Geometry check sheet. Reference: the model listing, model coordinates, mm. A direction names the side the tool comes from. Coordinates: 2 decimals unless noted, no trailing zeros. Loops run counter-clockwise (first coordinate to the right, second up) from the corner with the lowest first, then second, coordinate; pieces in that order, holes last.
from build123d import *

# Parameters (mm, degrees)
EXTRUDE_1_DEPTH     = 2
CUT_EXTRUDE_1_REACH = 72.175
SKETCH_2_R          = 1.3
CUT_EXTRUDE_2_REACH = 72.175
SKETCH_3_R          = 1.3
CUT_EXTRUDE_3_REACH = 72.175


with BuildPart() as part:
    # 草图1 → 凸台-拉伸1 (new body)
    with BuildSketch(Plane.XZ.offset(19.39)):
        Polygon((-51.8, -40.295836944), (-44.795836944, -47.3), (37.795836944, -47.3), (44.8, -40.295836944), (44.8, 27.295836944), (37.795836944, 34.3), (-44.795836944, 34.3), (-51.8, 27.295836944), align=None)
    extrude(amount=EXTRUDE_1_DEPTH)

    # 草图2 → 切除-拉伸1 (cut, up to next)
    with BuildSketch(Plane.XZ.offset(21.39), mode=Mode.PRIVATE) as cut_extrude_1_sk1:
        with Locations(Location((-39.011567772, -24.5, 0), (0, 0, 270))):
            Circle(SKETCH_2_R)
    cut_extrude_1_tool1 = extrude(cut_extrude_1_sk1.sketch, amount=-CUT_EXTRUDE_1_REACH, mode=Mode.PRIVATE) & part.part
    # 草图2 → 切除-拉伸1 (cut, up to next)
    with BuildSketch(Plane.XZ.offset(21.39), mode=Mode.PRIVATE) as cut_extrude_1_sk2:
        with Locations(Location((19, -24.5, 0), (0, 0, 270))):
            Circle(SKETCH_2_R)
    cut_extrude_1_tool2 = extrude(cut_extrude_1_sk2.sketch, amount=-CUT_EXTRUDE_1_REACH, mode=Mode.PRIVATE) & part.part
    # 草图2 → 切除-拉伸1 (cut, up to next)
    with BuildSketch(Plane.XZ.offset(21.39), mode=Mode.PRIVATE) as cut_extrude_1_sk3:
        with Locations(Location((-39.011567772, 24.535212594, 0), (0, 0, 270))):
            Circle(SKETCH_2_R)
    cut_extrude_1_tool3 = extrude(cut_extrude_1_sk3.sketch, amount=-CUT_EXTRUDE_1_REACH, mode=Mode.PRIVATE) & part.part
    # 草图2 → 切除-拉伸1 (cut, up to next)
    with BuildSketch(Plane.XZ.offset(21.39), mode=Mode.PRIVATE) as cut_extrude_1_sk4:
        with Locations(Location((19, 24.535212594, 0), (0, 0, 270))):
            Circle(SKETCH_2_R)
    cut_extrude_1_tool4 = extrude(cut_extrude_1_sk4.sketch, amount=-CUT_EXTRUDE_1_REACH, mode=Mode.PRIVATE) & part.part
    add(cut_extrude_1_tool1.solids().sort_by_distance((-39.011568, -21.39, -24.5))[0], mode=Mode.SUBTRACT)
    add(cut_extrude_1_tool2.solids().sort_by_distance((19, -21.39, -24.5))[0], mode=Mode.SUBTRACT)
    add(cut_extrude_1_tool3.solids().sort_by_distance((-39.011568, -21.39, 24.535213))[0], mode=Mode.SUBTRACT)
    add(cut_extrude_1_tool4.solids().sort_by_distance((19, -21.39, 24.535213))[0], mode=Mode.SUBTRACT)

    # 草图3 → 切除-拉伸2 (cut, up to next)
    with BuildSketch(Plane.XZ.offset(21.39), mode=Mode.PRIVATE) as cut_extrude_2_sk1:
        with Locations(Location((32, -44.5, 0), (0, 0, 270))):
            Circle(SKETCH_3_R)
    cut_extrude_2_tool1 = extrude(cut_extrude_2_sk1.sketch, amount=-CUT_EXTRUDE_2_REACH, mode=Mode.PRIVATE) & part.part
    # 草图3 → 切除-拉伸2 (cut, up to next)
    with BuildSketch(Plane.XZ.offset(21.39), mode=Mode.PRIVATE) as cut_extrude_2_sk2:
        with Locations(Location((-39, -44.5, 0), (0, 0, 270))):
            Circle(SKETCH_3_R)
    cut_extrude_2_tool2 = extrude(cut_extrude_2_sk2.sketch, amount=-CUT_EXTRUDE_2_REACH, mode=Mode.PRIVATE) & part.part
    # 草图3 → 切除-拉伸2 (cut, up to next)
    with BuildSketch(Plane.XZ.offset(21.39), mode=Mode.PRIVATE) as cut_extrude_2_sk3:
        with Locations(Location((32, 31.5, 0), (0, 0, 270))):
            Circle(SKETCH_3_R)
    cut_extrude_2_tool3 = extrude(cut_extrude_2_sk3.sketch, amount=-CUT_EXTRUDE_2_REACH, mode=Mode.PRIVATE) & part.part
    # 草图3 → 切除-拉伸2 (cut, up to next)
    with BuildSketch(Plane.XZ.offset(21.39), mode=Mode.PRIVATE) as cut_extrude_2_sk4:
        with Locations(Location((-39, 31.5, 0), (0, 0, 270))):
            Circle(SKETCH_3_R)
    cut_extrude_2_tool4 = extrude(cut_extrude_2_sk4.sketch, amount=-CUT_EXTRUDE_2_REACH, mode=Mode.PRIVATE) & part.part
    add(cut_extrude_2_tool1.solids().sort_by_distance((32, -21.39, -44.5))[0], mode=Mode.SUBTRACT)
    add(cut_extrude_2_tool2.solids().sort_by_distance((-39, -21.39, -44.5))[0], mode=Mode.SUBTRACT)
    add(cut_extrude_2_tool3.solids().sort_by_distance((32, -21.39, 31.5))[0], mode=Mode.SUBTRACT)
    add(cut_extrude_2_tool4.solids().sort_by_distance((-39, -21.39, 31.5))[0], mode=Mode.SUBTRACT)

    # 草图4 → 切除-拉伸3 (cut, up to next)
    with BuildSketch(Plane.XZ.offset(21.39), mode=Mode.PRIVATE) as cut_extrude_3_sk1:
        with BuildLine():
            Line((-40.69671065, 11.402772719), (-35.182847057, 19.74527284))
            ThreePointArc((-35.182847057, 19.74527284), (-32.411574314, 20.311000146), (-31.845847008, 17.539727403))
            Line((-31.845847008, 17.539727403), (-37.359710601, 9.197227281))
            ThreePointArc((-37.359710601, 9.197227281), (-40.130983344, 8.631499976), (-40.69671065, 11.402772719))
        make_face()
    cut_extrude_3_tool1 = extrude(cut_extrude_3_sk1.sketch, amount=-CUT_EXTRUDE_3_REACH, mode=Mode.PRIVATE) & part.part
    # 草图4 → 切除-拉伸3 (cut, up to next)
    with BuildSketch(Plane.XZ.offset(21.39), mode=Mode.PRIVATE) as cut_extrude_3_sk2:
        with BuildLine():
            Line((-32.69671065, 11.402772719), (-27.182847057, 19.74527284))
            ThreePointArc((-27.182847057, 19.74527284), (-24.411574314, 20.311000146), (-23.845847008, 17.539727403))
            Line((-23.845847008, 17.539727403), (-29.359710601, 9.197227281))
            ThreePointArc((-29.359710601, 9.197227281), (-32.130983344, 8.631499976), (-32.69671065, 11.402772719))
        make_face()
    cut_extrude_3_tool2 = extrude(cut_extrude_3_sk2.sketch, amount=-CUT_EXTRUDE_3_REACH, mode=Mode.PRIVATE) & part.part
    # 草图4 → 切除-拉伸3 (cut, up to next)
    with BuildSketch(Plane.XZ.offset(21.39), mode=Mode.PRIVATE) as cut_extrude_3_sk3:
        with BuildLine():
            Line((-24.69671065, 11.402772719), (-19.182847057, 19.74527284))
            ThreePointArc((-19.182847057, 19.74527284), (-16.411574314, 20.311000146), (-15.845847008, 17.539727403))
            Line((-15.845847008, 17.539727403), (-21.359710601, 9.197227281))
            ThreePointArc((-21.359710601, 9.197227281), (-24.130983344, 8.631499976), (-24.69671065, 11.402772719))
        make_face()
    cut_extrude_3_tool3 = extrude(cut_extrude_3_sk3.sketch, amount=-CUT_EXTRUDE_3_REACH, mode=Mode.PRIVATE) & part.part
    # 草图4 → 切除-拉伸3 (cut, up to next)
    with BuildSketch(Plane.XZ.offset(21.39), mode=Mode.PRIVATE) as cut_extrude_3_sk4:
        with BuildLine():
            Line((-16.69671065, 11.402772719), (-11.182847057, 19.74527284))
            ThreePointArc((-11.182847057, 19.74527284), (-8.411574314, 20.311000146), (-7.845847008, 17.539727403))
            Line((-7.845847008, 17.539727403), (-13.359710601, 9.197227281))
            ThreePointArc((-13.359710601, 9.197227281), (-16.130983344, 8.631499976), (-16.69671065, 11.402772719))
        make_face()
    cut_extrude_3_tool4 = extrude(cut_extrude_3_sk4.sketch, amount=-CUT_EXTRUDE_3_REACH, mode=Mode.PRIVATE) & part.part
    # 草图4 → 切除-拉伸3 (cut, up to next)
    with BuildSketch(Plane.XZ.offset(21.39), mode=Mode.PRIVATE) as cut_extrude_3_sk5:
        with BuildLine():
            Line((-8.69671065, 11.402772719), (-3.182847057, 19.74527284))
            ThreePointArc((-3.182847057, 19.74527284), (-0.411574314, 20.311000146), (0.154152992, 17.539727403))
            Line((0.154152992, 17.539727403), (-5.359710601, 9.197227281))
            ThreePointArc((-5.359710601, 9.197227281), (-8.130983344, 8.631499976), (-8.69671065, 11.402772719))
        make_face()
    cut_extrude_3_tool5 = extrude(cut_extrude_3_sk5.sketch, amount=-CUT_EXTRUDE_3_REACH, mode=Mode.PRIVATE) & part.part
    # 草图4 → 切除-拉伸3 (cut, up to next)
    with BuildSketch(Plane.XZ.offset(21.39), mode=Mode.PRIVATE) as cut_extrude_3_sk6:
        with BuildLine():
            Line((-0.69671065, 11.402772719), (4.817152943, 19.74527284))
            ThreePointArc((4.817152943, 19.74527284), (7.588425686, 20.311000146), (8.154152992, 17.539727403))
            Line((8.154152992, 17.539727403), (2.640289399, 9.197227281))
            ThreePointArc((2.640289399, 9.197227281), (-0.130983344, 8.631499976), (-0.69671065, 11.402772719))
        make_face()
    cut_extrude_3_tool6 = extrude(cut_extrude_3_sk6.sketch, amount=-CUT_EXTRUDE_3_REACH, mode=Mode.PRIVATE) & part.part
    add(cut_extrude_3_tool1.solids().sort_by_distance((-36.271279, -21.39, 14.47125))[0], mode=Mode.SUBTRACT)
    add(cut_extrude_3_tool2.solids().sort_by_distance((-28.271279, -21.39, 14.47125))[0], mode=Mode.SUBTRACT)
    add(cut_extrude_3_tool3.solids().sort_by_distance((-20.271279, -21.39, 14.47125))[0], mode=Mode.SUBTRACT)
    add(cut_extrude_3_tool4.solids().sort_by_distance((-12.271279, -21.39, 14.47125))[0], mode=Mode.SUBTRACT)
    add(cut_extrude_3_tool5.solids().sort_by_distance((-4.271279, -21.39, 14.47125))[0], mode=Mode.SUBTRACT)
    add(cut_extrude_3_tool6.solids().sort_by_distance((3.728721, -21.39, 14.47125))[0], mode=Mode.SUBTRACT)


solid = part.part
1) Access from +Z, -Z, +X, -X, +Y, -Y to the whole of each face (thin tool, end or side, straight path). Record for faces 1 (the flat face through (-4, -19.39, -6)), 2 (the flat face through (5.44, -20.4, 13.43)).
Data:
face 1: +Z, -Z, +X, -X, +Y
face 2: +Y, -Y
2) Depth check by flat-ended pin: pin 1 (2 mm diameter, centred on x = -39.01, z = 24.54, fed in from -Y); pin 2 (4 mm diameter, centred on x = -39.01, z = -24.5, fed in from +Y). Enter the tip coordinate at first touch or a pass-through.
Data:
pin 1: passes through
pin 2: stops at y = -19.39
3) Section check C-C on z = -44.5. Record the cut outline in (x, y).
Data:
outline: (-47.6, -21.39) - (-40.3, -21.39) - (-40.3, -19.39) - (-47.6, -19.39) - close; (-37.7, -21.39) - (30.7, -21.39) - (30.7, -19.39) - (-37.7, -19.39) - close; (33.3, -21.39) - (40.6, -21.39) - (40.6, -19.39) - (33.3, -19.39) - close
4) Section check B-B on z = 13. Record the cut outline in (x, y), and give its area (3 significant figures).
Data:
outline: (-51.8, -21.39) - (-39.64, -21.39) - (-39.64, -19.39) - (-51.8, -19.39) - close; (-34.85, -21.39) - (-31.64, -21.39) - (-31.64, -19.39) - (-34.85, -19.39) - close; (-26.85, -21.39) - (-23.64, -21.39) - (-23.64, -19.39) - (-26.85, -19.39) - close; (-18.85, -21.39) - (-15.64, -21.39) - (-15.64, -19.39) - (-18.85, -19.39) - close; (-10.85, -21.39) - (-7.64, -21.39) - (-7.64, -19.39) - (-10.85, -19.39) - close; (-2.85, -21.39) - (0.36, -21.39) - (0.36, -19.39) - (-2.85, -19.39) - close; (5.15, -21.39) - (44.8, -21.39) - (44.8, -19.39) - (5.15, -19.39) - close
area: 136 mm2
5) Mould release check, pull along X, two halves, no side actions. Record for faces 3 (the flat face through (41.347, -20.376, 30.749)), 4 (the cylindrical face through (-40.094, -20.404, 8.608)), 5 (the flat face through (-51.8, -20, -6)): +X half, -X half, draft (parallel to the pull), parting line (faces both ways), or undercut.
Data:
face 3: +X half
face 4: undercut
face 5: -X half
6) Material ranges on probe 1 along X at (y, z) = (-20.4, -24.5); probe 2 along Z at (x, y) = (-39.5, -20.7); probe 3 along X at (y, z) = (-20.55, 31.5), recorded low to high.
Data:
probe 1: x = -51.8 to -40.31, -37.71 to 17.7, 20.3 to 44.8
probe 2: z = -47.3 to -45.7, -43.3 to -25.7, -23.3 to 8.36, 13.21 to 23.33, 25.74 to 30.3, 32.7 to 34.3
probe 3: x = -47.6 to -40.3, -37.7 to 30.7, 33.3 to 40.6
7) Section check A-A on x = 19. Record the cut outline in (y, z), and give its area (3 significant figures).
Data:
outline: (-21.39, -47.3) - (-19.39, -47.3) - (-19.39, -25.8) - (-21.39, -25.8) - close; (-21.39, -23.2) - (-19.39, -23.2) - (-19.39, 23.24) - (-21.39, 23.24) - close; (-21.39, 25.84) - (-19.39, 25.84) - (-19.39, 34.3) - (-21.39, 34.3) - close
area: 153 mm2
8) Section check D-D on y = -20. Count the separate pieces of the cut face and the enclosed holes in it, and give its area (3 significant figures).
Data:
separate pieces: 1
enclosed holes: 14
area: 7,430 mm2
